Geometry check sheet. Reference: the model listing, model coordinates, mm. A direction names the side the tool comes from. Round coordinates to 2 decimals unless told otherwise and drop trailing zeros. Write each loop counter-clockwise with the first axis right and the second up, starting at its lowest first coordinate (ties: lowest second). Pieces come first, ordered by that corner, then holes. Notation, with made-up numbers: (11.5, -34) - (59.5, -34) arc R22 ccw to (59.5, 0) - close; hole circle Ø2 at (4.25, 62.25). An arc over 180 degrees is marked (long way). Return JSON: item names as keys, results as strings.
Autodesk Inventor part; units mm, degrees
ref_plane "Work Plane1" through (-88.9, 162.0885, -255.3455) normal (0, -0.8660254, -0.5) x (1, 0, 0)
ref_plane "YZ Plane" through (0, 0, 0) normal (1, 0, 0) x (0, 1, 0)
ref_plane "XZ Plane" through (0, 0, 0) normal (0, 1, 0) x (-1, 0, 0)
sketch "Sketch1" plane through (0, 0, 0) normal (1, 0, 0) x (0, 1, 0)
  arc A0 (0, -277.0467) -> (178.0822, -212.2301) centre (0, 0) ccw
  arc A1 (0, -302.4467) -> (194.409, -231.6876) centre (0, 0) ccw
  line L0 (178.0822, -212.2301) -> (194.409, -231.6876)
  line L1 (0, -277.0467) -> (0, -302.4467)
  line L2 (168.1662, -220.1704) -> (184.6802, -239.851)
  line L3 (184.6802, -239.851) -> (204.1378, -223.5242)
  line L4 (204.1378, -223.5242) -> (187.811, -204.0667)
  line L5 (187.811, -204.0667) -> (168.3534, -220.3935)
  line L6 (168.3534, -220.3935) -> (204.1378, -223.5242) construction
  line L7 (184.6802, -239.851) -> (187.811, -204.0667) construction
  arc A2 (0, -277.0467) -> (138.5234, -239.9295) centre (0, 0) ccw
  line L8 (138.5234, -239.9295) -> (151.2234, -261.9266)
  line L9 (162.2219, -255.5766) -> (140.2248, -268.2766)
  line L10 (140.2248, -268.2766) -> (127.3792, -246.0273)
  line L11 (127.5248, -246.2795) -> (149.5219, -233.5795)
  line L12 (149.5219, -233.5795) -> (162.2219, -255.5766)
  line L13 (162.2219, -255.5766) -> (127.5248, -246.2795) construction
  line L14 (140.2248, -268.2766) -> (149.5219, -233.5795) construction
  point P0 (186.2456, -221.9589)
  point P1 (184.5088, -239.6467)
  point P2 (144.8734, -250.928)
  point P3 (140.0915, -268.0455)
  dimension "d1" = 277.0467
  dimension "d2" = 40
  dimension "d4" = 25.4
  dimension "d5" = 25.4
  dimension "d32" = 30
  dimension "d33" = 25.4
extrude "Extrusion1" add sketch "Sketch1" along normal mid plane 177.8 contours A0 L11 L10 | L11 L12 A1 L8 | L8 A1 L10 L11 | A0 L2 A1 L12 L11
sketch "Sketch3" plane through (-88.9, 168.1662, -220.1704) normal (0, 0.7660444, 0.6427876) x (1, 0, 0)
  line L0 (88.9, 0) -> (88.9, 25.6912)
  line L1 (177.8, 25.4245) -> (177.8, 0)
  point P0 (88.9, -276.7555)
  point P1 (152.4, 12.9912)
  dimension "d17" = 25.4
  dimension "d18" = 12.7
hole "Hole2" at (63.5, 176.5168, -230.1223) direction (0, -0.7660444, -0.6427876) diameter 4.445 depth 38.1 counterbore diameter 5.588 counterbore depth 8.255
pattern_linear "Rectangular Pattern2" count 3 spacing 50.8 along (-1, 0, 0) of "Hole2"
sketch "Sketch5" plane through (-88.9, 140.2248, -268.2766) normal (0, -0.8660254, -0.5) x (1, 0, 0)
  point P0 (88.9, 302.4467)
sketch "Sketch6" plane through (-88.9, 140.2248, -268.2766) normal (0, -0.8660254, -0.5) x (1, 0, 0)
  line L0 (0, 0.2668) -> (0, 25.6912)
  line L1 (0, 25.6912) -> (177.8, 25.6912)
  point P0 (88.9, 302.4467)
  point P1 (25.4, 12.7)
  dimension "d50" = 25.4
  dimension "d51" = 12.9912
hole "Hole3" at (-63.5, 133.8748, -257.278) direction (0, 0.8660254, 0.5) diameter 4.445 end through all
ref_plane "Work Plane1" through (-88.9, 162.0885, -255.3455) normal (0, -0.8660254, -0.5) x (1, 0, 0)
sketch "Sketch7" plane through (-88.9, 162.0885, -255.3455) normal (0, -0.8660254, -0.5) x (1, 0, 0)
  circle A0 centre (25.4, 12.4332) radius 2.2225
  circle A1 centre (25.4, 12.4332) radius 4.064
  point P0 (88.9, 302.18)
  dimension "d44" = 8.128
extrude "Extrusion2" cut sketch "Sketch7" against normal through all contours A0 | A1
pattern_linear "Rectangular Pattern3" count 3 spacing 50.8 along (1, 0, 0) of "Extrusion2", "Hole3"
properties part number "HoodBraceExtension"
(1) Gauge pin test, flat ends, axial feed: pin 1 (4 mm diameter, centred on x = 23.5, y = 175.5, fed in from -Z); pin 2 (5 mm diameter, centred on x = -6.5, y = 150, fed in from +Z); pin 3 (1 mm diameter, centred on x = -40, z = -250.5, fed in from +Y). Record the tip position at first contact, or that the pin passes through.
Response values:
{"pin 1": "stops at z = -247.73", "pin 2": "stops at z = -231.3", "pin 3": "stops at y = 170.22"}
(2) Section check A-A, the plane x = -76. Enter the section's corners in (y, z), plus the area to 3 significant figures.
Response values:
{"outline": "(127.38, -246.03) - (140.09, -268.05) arc R302.45 ccw to (184.51, -239.65) - (168.17, -220.17) arc R277.05 cw to start", "area": "1,280 mm^2"}
(3) Access from +Z, -Z, +X, -X, +Y, -Y to the whole of each face (thin tool, end or side, straight path). Record for faces 1 (the face through (-1.24, 176.22, -229.77)), 2 (the face through (-38.13, 147.31, -254.59)).
Response values:
{"face 1": "+Z, +X, -X, +Y", "face 2": "none"}
(4) Material ranges on line 1 along Y through (x, z) = (-62, -251); line 2 along Y through (x, z) = (-15, -245); line 3 along Z through (x, y) = (9, 170.5), recorded low to high. Write a range as [from, to].
Response values:
{"line 1": "y = [130.25, 141.47], [148.03, 168.74]", "line 2": "y = [129.34, 156.12], [161.84, 177.34]", "line 3": "z = [-249.81, -222.95]"}
(5) Section check C-C, the plane y = 160.5. Give the number of separate pieces and of enclosed holes in the cut face, plus the area to 3 significant figures.
Response values:
{"separate pieces": "1", "enclosed holes": "6", "area": "5,190 mm^2"}
(6) Release check for a two-part mould opening along Y. For faces 3 (the face through (-39.602, 159.655, -246.41)), 4 (the face through (-1.245, 163.231, -254.617)), 5 (the face through (-1.24, 148.62, -233.81)) record: pulls with the +Y half, pulls with the -Y half, needs draft (parallel to the pull), parting line crosses it, or undercut.
Response values:
{"face 3": "undercut", "face 4": "pulls with the +Y half", "face 5": "pulls with the -Y half"}
(7) Section check B-B, the plane z = -264.5. Enter the section's corners in (x, y).
Response values:
{"outline": "(-88.9, 138.04) - (88.9, 138.04) - (88.9, 146.68) - (-88.9, 146.68) - close"}
